```python
from build123d import *

# Parameters (mm, degrees)
F1_DEPTH = 7
F2_R     = 1.65
F3_DEPTH = 9.001


with BuildPart() as f1:
    # F0 (on Top) → F1 (new body)
    with BuildSketch(Plane.XY):
        with BuildLine():
            ThreePointArc((0, 3.1), (2.192031, 2.192031), (3.1, 0))
            Line((3.1, 0), (3.1, -3.1))
            Line((3.1, -3.1), (15, -3.1))
            Line((15, -3.1), (15, 5.9))
            Line((15, 5.9), (0, 5.9))
            Line((0, 5.9), (-15, 5.9))
            Line((-15, 5.9), (-15, -3.1))
            Line((-15, -3.1), (-3.1, -3.1))
            Line((-3.1, -3.1), (-3.1, 0))
            ThreePointArc((-3.1, 0), (-2.192031, 2.192031), (0, 3.1))
        make_face()
    extrude(amount=F1_DEPTH)

    # F2 (on face) → F3 (cut, through all)
    with BuildSketch(Plane(origin=(0, 5.9, 0), x_dir=(-1, 0, 0), z_dir=(0, 1, 0))):
        with Locations((11.3, 3.5)):
            Circle(F2_R)
        with Locations((-11.3, 3.5)):
            Circle(F2_R)
    extrude(amount=-F3_DEPTH, mode=Mode.SUBTRACT)


solid = f1.part
```
Input: part model. Units: mm. Frame: model coordinates. A direction names the side the tool comes from. Round coordinates to 2 decimals unless told otherwise and drop trailing zeros. Loops run counter-clockwise (first coordinate to the right, second up) from the corner with the lowest first, then second, coordinate; pieces in that order, holes last.
1) Material intervals for line 1 (X direction, y = -0.5, z = 5); line 2 (X direction, y = -1.25, z = 4.5); line 3 (Z direction, x = 11.3, y = 1.75), sorted ascending.
Ans:
line 1: x = -15 to -11.99, -10.61 to -3.1, 3.1 to 10.61, 11.99 to 15
line 2: x = -15 to -12.61, -9.99 to -3.1, 3.1 to 9.99, 12.61 to 15
line 3: z = 0 to 1.85, 5.15 to 7
2) Section query B-B on x = -11.3. Return the cut outline in (y, z).
Ans:
outline: (-3.1, 0) - (5.9, 0) - (5.9, 1.85) - (-3.1, 1.85) - close; (-3.1, 5.15) - (5.9, 5.15) - (5.9, 7) - (-3.1, 7) - close
3) Pull-direction query (X, two-part tool) for faces 3 (the flat face through (-0.2, 3.5, 7)), 4 (the flat face through (-3.1, -2, 3)), 5 (the flat face through (-15, 1, 3)); classes: released by +X, released by -X, zero draft, split by the parting line, or undercut.
Ans:
face 3: zero draft
face 4: undercut
face 5: released by -X
4) Pin query (flat end, axial travel): pin 1 (3 mm diameter, centred on x = -11.3, z = 3.5, fed in from +Y); pin 2 (2 mm diameter, centred on x = -1, z = 3, fed in from -Y). Return the tip coordinate at first contact, or that it passes through.
Ans:
pin 1: passes through
pin 2: stops at y = 2.37
5) Section query D-D on z = 6.25. Return the cut outline in (x, y).
Ans:
outline: (-15, -3.1) - (-3.1, -3.1) - (-3.1, 0) arc R3.1 cw to (3.1, 0) - (3.1, -3.1) - (15, -3.1) - (15, 5.9) - (-15, 5.9) - close
6) Section query A-A on y = -1. Return the cut outline in (x, z), plus the area to 3 significant figures.
Ans:
outline: (-15, 0) - (-3.1, 0) - (-3.1, 7) - (-15, 7) - close; (3.1, 0) - (15, 0) - (15, 7) - (3.1, 7) - close; hole circle Ø3.3 at (-11.3, 3.5); hole circle Ø3.3 at (11.3, 3.5)
area: 149 mm2
7) Section query C-C on z = 3.5. Return the cut outline in (x, y), plus the area to 3 significant figures.
Ans:
outline: (-15, -3.1) - (-12.95, -3.1) - (-12.95, 5.9) - (-15, 5.9) - close; (-9.65, -3.1) - (-3.1, -3.1) - (-3.1, 0) arc R3.1 cw to (3.1, 0) - (3.1, -3.1) - (9.65, -3.1) - (9.65, 5.9) - (-9.65, 5.9) - close; (12.95, -3.1) - (15, -3.1) - (15, 5.9) - (12.95, 5.9) - close
area: 176 mm2
8) Set-up query: faces 1 (the flat face through (3.1, -2, 3)), 2 (the flat face through (0, 5.9, 3)). Return all of +Z, -Z, +X, -X, +Y, -Y with unobstructed straight access to the full face (end or side cutting, diameter ignored); none if empty.
Ans:
face 1: +Z, -Z, -Y
face 2: +Z, -Z, +X, -X, +Y
